Design review of the part built by this model. Coordinates are the model's own, in mm. A direction names the side the tool comes from. Coordinates: 2 decimals unless noted, no trailing zeros. Write each loop counter-clockwise with the first axis right and the second up, starting at its lowest first coordinate (ties: lowest second). Pieces come first, ordered by that corner, then holes. Notation, with made-up numbers: (83, 39.5) - (90, 39.5) arc R16 cw to (90, 58.5) - close; hole circle Ø4 at (60, -37.5). An arc over 180 degrees is marked (long way). Answer as a JSON object with one key per item and string values.
Autodesk Inventor part; units mm, degrees
ref_plane "YZ Plane" through (0, 0, 0) normal (1, 0, 0) x (0, 1, 0)
ref_plane "XZ Plane" through (0, 0, 0) normal (0, 1, 0) x (-1, 0, 0)
ref_plane "XY Plane" through (0, 0, 0) normal (0, 0, 1) x (1, 0, 0)
sketch "Skizze1" plane through (0, 0, 0) normal (0, 0, 1) x (1, 0, 0)
  circle A0 centre (0, 0) radius 12.5
  dimension "d0" = 25
extrude "Extrusion1" add sketch "Skizze1" along normal blind 86
sketch "Skizze3" plane through (0, 0, 86) normal (0, 0, 1) x (1, 0, 0)
  circle A0 centre (0, 0) radius 12.5
  line L0 (-12.5, 0) -> (12.5, 0)
  line L1 (12.5, 0) -> (12.5, -35)
  line L2 (12.5, -35) -> (-12.5, -35)
  line L3 (-12.5, -35) -> (-12.5, 0)
  dimension "d4" = 35
extrude "Extrusion2" add sketch "Skizze3" against normal blind 75 contours L1 L2 L3 A0
sketch "Skizze4" plane through (0, 0, 86) normal (0, 0, 1) x (1, 0, 0)
  line L0 (-4.1, -35.0592) -> (4.1, -35.0592)
  line L1 (4.1, -35.0592) -> (4.1, -0.0592)
  line L2 (4.1, -0.0592) -> (-4.1, -0.0592)
  line L3 (-4.1, -0.0592) -> (-4.1, -35.0592)
  line L4 (-12.5, 0) -> (-12.5, -35)
  line L5 (12.5, -35) -> (12.5, 0)
  point P0 (0, 0)
  dimension "d7" = 8.2
  dimension "d8" = 35
  dimension "d9" = 8.4
  dimension "d10" = 8.4
extrude "Extrusion3" cut sketch "Skizze4" against normal up to surface (75 mm away)
sketch "Skizze5" plane through (0, 0, 0) normal (0, 0, -1) x (-1, 0, 0)
  line L0 (-4.05, 11.8427) -> (4.05, 11.8427)
  line L1 (4.05, 11.8427) -> (4.05, -11.8427)
  line L2 (4.05, -11.8427) -> (-4.05, -11.8427)
  line L3 (-4.05, -11.8427) -> (-4.05, 11.8427)
  circle A0 centre (0, 0) radius 12.5
  point P0 (4.05, -11.8257)
  point P1 (4.05, 11.8257)
  point P2 (-4.05, 11.8257)
  point P3 (-4.05, -11.8257)
  dimension "d13" = 8.1
  dimension "d14" = 4.05
  dimension "d16" = 25
extrude "Extrusion4" add sketch "Skizze5" along normal blind 10 contours L3 A0 | A0 L1
sketch "Skizze6" plane through (4.05, -11.8257, 0) normal (-1, 0, 0) x (0, 0, 1)
  circle A0 centre (-5, 8) radius 2.525
  line L0 (-10, 23.6514) -> (-10, 0)
  circle A1 centre (-5, 15.6514) radius 2.525
  line L1 (0, 23.6514) -> (-10, 23.6514)
  line L2 (0, 0) -> (-10, 0)
  point P0 (0, 11.8257)
  dimension "d19" = 5.05
  dimension "d20" = 5
  dimension "d21" = 5.05
  dimension "d22" = 0
  dimension "d23" = 8
  dimension "d24" = 8
  dimension "d25" = 7.6514
extrude "Extrusion5" cut sketch "Skizze6" along normal mid plane 500
sketch "Skizze7" plane through (12.5, -35, 86) normal (1, 0, 0) x (0, 0, -1)
  circle A0 centre (55, 24) radius 2.5
  circle A1 centre (15, 24) radius 2.5
  circle A2 centre (15, 10) radius 2.5
  circle A3 centre (55, 10) radius 2.5
  line L0 (0, 0) -> (0, 35)
  line L1 (0, 0) -> (75, 0)
  line L2 (75, 35) -> (0, 35)
  point P0 (86, 35)
  dimension "d28" = 5
  dimension "d29" = 5
  dimension "d30" = 5
  dimension "d31" = 5
  dimension "d32" = 15
  dimension "d33" = 15
  dimension "d34" = 40
  dimension "d35" = 40
  dimension "d36" = 0
  dimension "d37" = 10
  dimension "d38" = 14
  dimension "d39" = 14
  dimension "d42" = 11
extrude "Extrusion6" cut sketch "Skizze7" against normal up to surface (25 mm away)
properties part number "Fahnenhalter"
(1) Tool access review of faces 4 (the face through (4.05, 0, -5)), 5 (the face through (-4.1, -17, 49)), 6 (the face through (5, -11, 86)): name each direction out of +Z, -Z, +X, -X, +Y, -Y from which nothing blocks a thin tool from reaching the whole face with its end or side.
Solved:
{"face 4": "-Z, +Y, -Y", "face 5": "+Z, -Y", "face 6": "+Z, +X, -X, +Y, -Y"}
(2) Take a section at B-B, the plane y = -25. Write out the cut boundary in (x, z), and give its area (3 significant figures).
Solved:
{"outline": "(-12.5, 11) - (-4.1, 11) - (-4.1, 28.5) - (-12.5, 28.5) - close; (-12.5, 33.5) - (-4.1, 33.5) - (-4.1, 68.5) - (-12.5, 68.5) - close; (-12.5, 73.5) - (-4.1, 73.5) - (-4.1, 86) - (-12.5, 86) - close; (4.1, 11) - (12.5, 11) - (12.5, 28.5) - (4.1, 28.5) - close; (4.1, 33.5) - (12.5, 33.5) - (12.5, 68.5) - (4.1, 68.5) - close; (4.1, 73.5) - (12.5, 73.5) - (12.5, 86) - (4.1, 86) - close", "area": "1,090 mm^2"}
(3) For pin 1 (3 mm diameter, centred on y = 5, z = -5.5, fed in from -X); pin 2 (6 mm diameter, centred on y = -3.83, z = -5, fed in from -X); pin 3 (3 mm diameter, centred on x = -5.5, y = -27.5, fed in from -Z), all flat-tipped, find the tip position at first contact; note any pin that passes through.
Solved:
{"pin 1": "stops at x = -11.25", "pin 2": "stops at x = -12.47", "pin 3": "stops at z = 11"}
(4) The part is to be moulded in two halves that separate along Z. For faces 1 (the face through (-12.5, -18, 49)), 2 (the face through (-8, -21, 11)), 3 (the face through (8.36, -13.44, 31.54)), say which applies: pulls with the +Z half, pulls with the -Z half, needs draft (parallel to the pull), parting line crosses it, or undercut.
Solved:
{"face 1": "needs draft", "face 2": "pulls with the -Z half", "face 3": "undercut"}
(5) Take a section at A-A, the plane z = 71. Write out the cut boundary in (x, y), and give its area (3 significant figures).
Solved:
{"outline": "(-12.5, -35) - (-4.1, -35) - (-4.1, -27.5) - (-12.5, -27.5) - close; (-12.5, -22.5) - (-4.1, -22.5) - (-4.1, -13.5) - (-12.5, -13.5) - close; (-12.5, -8.5) - (-4.1, -8.5) - (-4.1, -0.06) - (4.1, -0.06) - (4.1, -8.5) - (12.5, -8.5) - (12.5, 0) arc R12.5 ccw to (-12.5, 0) - close; (4.1, -35) - (12.5, -35) - (12.5, -27.5) - (4.1, -27.5) - close; (4.1, -22.5) - (12.5, -22.5) - (12.5, -13.5) - (4.1, -13.5) - close", "area": "666 mm^2"}
(6) Take a section at D-D, the plane x = 0. Write out the cut boundary in (y, z).
Solved:
{"outline": "(-12.5, 0) - (12.5, 0) - (12.5, 86) - (-0.06, 86) - (-0.06, 11) - (-12.5, 11) - close"}
(7) To check wall thickness, follow line 1 (X direction, y = -19.5, z = 50.5); line 2 (Z direction, x = -5.75, y = -27); line 3 (Y direction, x = 8.5, z = 71). State the ranges of each line that lie inside material, in increasing order. Write a range as from..to.
Solved:
{"line 1": "x = -12.5..-4.1, 4.1..12.5", "line 2": "z = 11..29.5, 32.5..69.5, 72.5..86", "line 3": "y = -35..-27.5, -22.5..-13.5, -8.5..9.17"}
(8) Take a section at C-C, the plane y = -18. Write out the cut boundary in (x, z), and give its area (3 significant figures).
Solved:
{"outline": "(-12.5, 11) - (-4.1, 11) - (-4.1, 86) - (-12.5, 86) - close; (4.1, 11) - (12.5, 11) - (12.5, 86) - (4.1, 86) - close", "area": "1,260 mm^2"}
